For this review, take the finished solid that the model builds, in its own axes (mm). A direction names the side the tool comes from. Give positions to 0.01 mm unless a question says otherwise; leave off trailing zeros. Write each loop counter-clockwise with the first axis right and the second up, starting at its lowest first coordinate (ties: lowest second). Pieces come first, ordered by that corner, then holes. Notation, with made-up numbers: M 12,-21 L 18,-21 A16 cw 18,7 Z; hole C 48,7.5 d2. An arc over 180 degrees is marked long. One line per item, written item: value. Start each with the question number.
Item 1: Consider section C-C, the plane y = -4.5. Write out the cut boundary in (x, z), and give its area (3 significant figures).
Item 2: Consider section A-A, the plane x = 0. Write out the cut boundary in (y, z).
Item 3: To check wall thickness, follow probe 1 along X at (y, z) = (7, -190); probe 2 along Z at (x, y) = (0, -7.75); probe 3 along Y at (x, z) = (14, -186.5). State the ranges of each line that lie inside material, in increasing order.
Item 4: Clearance check with flat-ended pins moving along their axes: pin 1 Ø8 at (x, y) = (1.5, -3.5) entering from -Z; pin 2 Ø2 at (x, y) = (0.5, -6) entering from +Z; pin 3 Ø1.5 at (x, z) = (-8.5, -175.5) entering from -Y. State where each tip first meets the part, or that it passes through.
Item 5: Mouldability with a two-part tool opening along Z and no side actions: class faces 1 (the face through (-3.38, 8.94, -205.19)), 2 (the face through (-4.48, -0.11, -210.15)) as released by +Z, released by -Z, zero draft, split by the parting line, or undercut.
Item 6: Consider section B-B, the plane y = 9.75. Write out the cut boundary in (x, z).
Item 7: Tool access review of faces 3 (the face through (0, 5.08, -190)), 4 (the face through (0, -5.08, -190)): name each direction out of +Z, -Z, +X, -X, +Y, -Y from which nothing blocks a thin tool from reaching the whole face with its end or side.
```python
from build123d import *

# Parameters (mm, degrees)
F4_R     = 20.6580157973
F5_DEPTH = 12.7
F6_DEPTH = 12.7
F7_R     = 5.08
F8_DEPTH = 7.62
F9_DEPTH = 7.62


# Not quite as in the source:
# - a feature of the source that left no trace in its solid (it failed there, or was rolled back) is left out


with BuildPart() as f5:
    # F4 (on Front) → F5 (new body)
    with BuildSketch(Plane.XZ):
        with Locations((0, -189.9833083153)):
            Circle(F4_R)
    extrude(amount=F5_DEPTH)

    # F6 (add): a face of the model
    f6_faces = [f5.faces().sort_by_distance(p)[0] for p in [
        (0, 0, -189.9833083153),
    ]]
    extrude(f6_faces, amount=F6_DEPTH)

    # F7
    f7_edges = [f5.edges().sort_by_distance(p)[0] for p in [
        (-20.658016, -12.7, -189.983308),
        (-20.658016, 12.7, -189.983308),
    ]]
    fillet(f7_edges, radius=F7_R)

    # F8 (cut): a face of the model
    f8_faces = [f5.faces().sort_by_distance(p)[0] for p in [
        (0, -12.7, -189.9833083153),
    ]]
    extrude(f8_faces, amount=-F8_DEPTH, mode=Mode.SUBTRACT)

    # F9 (cut): a face of the model
    f9_faces = [f5.faces().sort_by_distance(p)[0] for p in [
        (0, 12.7, -189.9833083153),
    ]]
    extrude(f9_faces, amount=-F9_DEPTH, mode=Mode.SUBTRACT)


solid = f5.part
```
Model answer:
1. outline: C 0,-189.98 d41.32
1. area: 1,340 mm2
2. outline: M -12.7,-205.56 A5.08 ccw -7.62,-210.64 L 7.62,-210.64 A5.08 ccw 12.7,-205.56 L 5.08,-205.56 L 5.08,-174.41 L 12.7,-174.41 A5.08 ccw 7.62,-169.33 L -7.62,-169.33 A5.08 ccw -12.7,-174.41 L -5.08,-174.41 L -5.08,-205.56 Z
3. probe 1: x = -20.66 to -15.58, 15.58 to 20.66
3. probe 2: z = -210.64 to -205.56, -174.41 to -169.33
3. probe 3: y = -5.08 to 5.08
4. pin 1: stops at z = -210.64
4. pin 2: stops at z = -169.33
4. pin 3: stops at y = -12.68
5. face 1: undercut
5. face 2: split by the parting line
6. outline: C 0,-189.98 d40.38; hole C 0,-189.98 d31.16
7. face 3: +Y
7. face 4: -Y
